The figure shows three views and two pictorial views of one solid part (mm, origin at its lowest corner). Answer the questions. Coordinates: 2 decimals unless noted, no trailing zeros. Loops run counter-clockwise (first coordinate to the right, second up) from the corner with the lowest first, then second, coordinate; pieces in that order, holes last. Notation, with made-up numbers: (-25, -7.5) - (14, -7.5) arc R10 cw to (14, 6.5) - close; hole circle Ø8 at (47.5, 78.5). An arc over 180 degrees is marked (long way). Return JSON: item names as keys, results as strings. Group by question number.
1. Section B-B (x = 16.5) is taken. Write down the section's boundary in (y, z), and give its area (3 significant figures).
2. Section A-A (y = 5.25) is taken. Write down the section's boundary in (x, z).
3. Find the intervals of material crossed by line 1 along Z through (x, y) = (17, 1) (1 decimal); line 2 along Z through (x, y) = (27, 1.5), in increasing order.
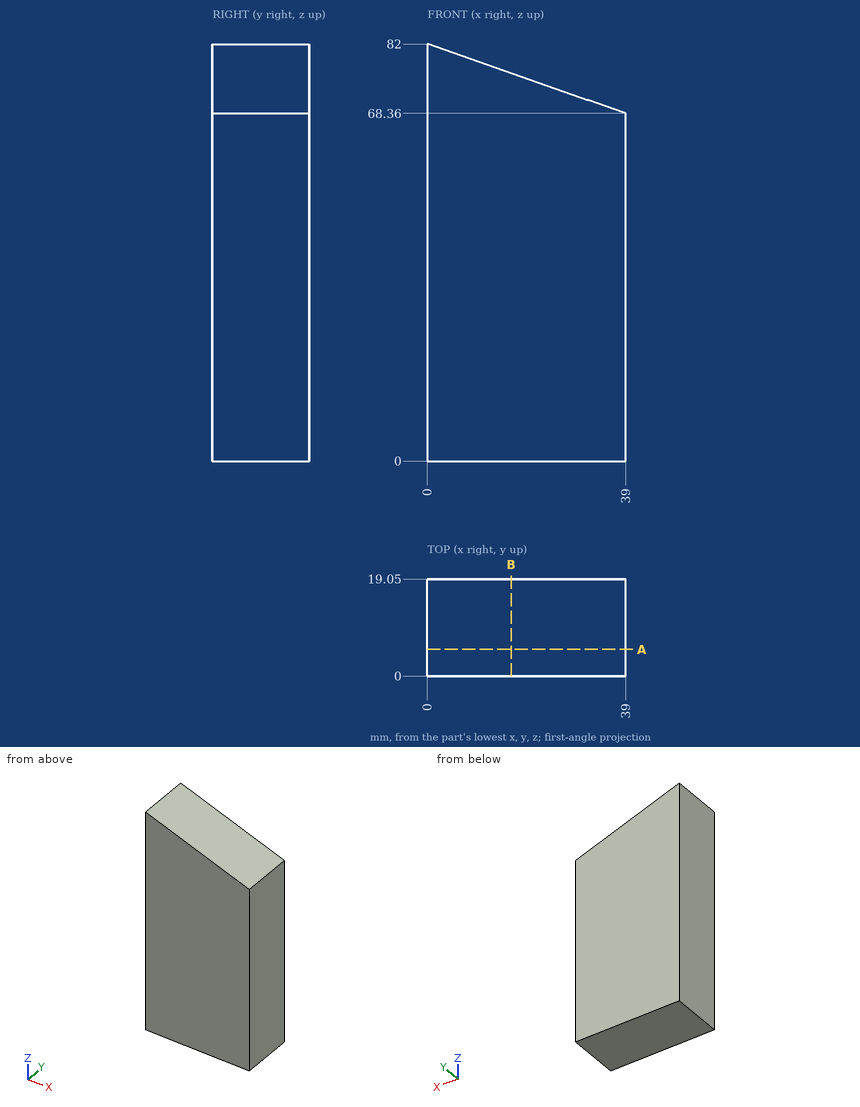
The answers:
{
 "1": {"outline": "(0, 0) - (19.05, 0) - (19.05, 76.23) - (0, 76.23) - close", "area": "1,450 mm2"},
 "2": {"outline": "(0, 0) - (39, 0) - (39, 68.36) - (0, 82) - close"},
 "3": {"line 1": "z = 0 to 76.1", "line 2": "z = 0 to 72.56"}
}
